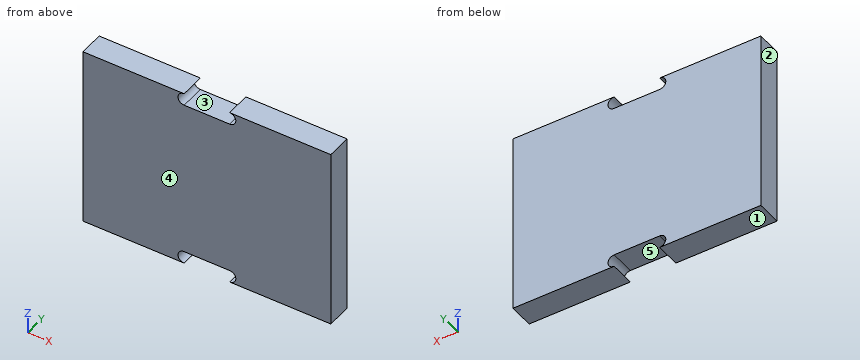
```python
from build123d import *

# Parameters (mm, degrees)
BOSS_EXTRUDE1_DEPTH = 6


with BuildPart() as part:
    # Sketch1 → Boss-Extrude1 (new body)
    with BuildSketch(Plane(origin=(0, 0, 0), x_dir=(1, 0, 0), z_dir=(0, 1, 0))):
        with BuildLine():
            Line((-30, 0), (-30, 22.2))
            Line((-30, 22.2), (-5.5, 22.2))
            ThreePointArc((-5.5, 22.2), (-7, 20.7), (-5.5, 19.2))
            Line((-5.5, 19.2), (0, 19.2))
            Line((0, 19.2), (5.5, 19.2))
            ThreePointArc((5.5, 19.2), (7, 20.7), (5.5, 22.2))
            Line((5.5, 22.2), (30, 22.2))
            Line((30, 22.2), (30, 0))
            Line((30, 0), (30, -22.2))
            Line((30, -22.2), (5.5, -22.2))
            ThreePointArc((5.5, -22.2), (7, -20.7), (5.5, -19.2))
            Line((5.5, -19.2), (0, -19.2))
            Line((0, -19.2), (-5.5, -19.2))
            ThreePointArc((-5.5, -19.2), (-7, -20.7), (-5.5, -22.2))
            Line((-5.5, -22.2), (-30, -22.2))
            Line((-30, -22.2), (-30, 0))
        make_face()
    extrude(amount=BOSS_EXTRUDE1_DEPTH)


solid = part.part
```
CAD build for the part. Positions are in the model's coordinates, mm. Face numbers are marked on the shaded views. A direction names the side the tool comes from. Coordinates: 2 decimals unless noted, no trailing zeros. Loops run counter-clockwise (first coordinate to the right, second up) from the corner with the lowest first, then second, coordinate; pieces in that order, holes last. Notation, with made-up numbers: (84, -16) - (101, -16) arc R16 cw to (101, -4) - close; hole circle Ø4 at (15.25, -34.75). An arc over 180 degrees is marked (long way). Return JSON: item names as keys, results as strings.
1. Drop flat-ended pins along their axis: pin 1 (1.5 mm diameter, centred on x = 2, z = 6.5, fed in from -Y); pin 2 (2 mm diameter, centred on x = 0, y = 2, fed in from +Z). Give the stop position or say it passes through.
Result:
{"pin 1": "stops at y = 0", "pin 2": "stops at z = 19.2"}
2. Probe L1, parallel to X at y = 0.55, z = 20.5; L2, parallel to Z at x = 6.5, y = 3.1; L3, parallel to Z at x = 3, y = 4.45. List the from-to ranges inside material, lowest first. Write a range as from..to.
Result:
{"L1": "x = -30..-6.99, 6.99..30", "L2": "z = -22.2..-21.82, -19.58..19.58, 21.82..22.2", "L3": "z = -19.2..19.2"}
3. Band-saw the part on A-A (z = 20.7). Give the cut face in (x, y).
Result:
{"outline": "(-30, 0) - (-7, 0) - (-7, 6) - (-30, 6) - close; (7, 0) - (30, 0) - (30, 6) - (7, 6) - close"}
4. Band-saw the part on C-C (x = 1.5). Give the cut face in (y, z).
Result:
{"outline": "(0, -19.2) - (6, -19.2) - (6, 19.2) - (0, 19.2) - close"}
5. 3-axis set-ups, long thin cutter, end or side, ignore diameter. For the marked faces 4 and 5: which of +Z, -Z, +X, -X, +Y, -Y reach the whole face in a straight line?
Result:
{"face 4": "+Z, -Z, +X, -X, -Y", "face 5": "-Z, +Y, -Y"}
6. Band-saw the part on B-B (y = 2.1). Give the cut face in (x, z), and give its area (3 significant figures).
Result:
{"outline": "(-30, -22.2) - (-5.5, -22.2) arc R1.5 cw to (-5.5, -19.2) - (5.5, -19.2) arc R1.5 cw to (5.5, -22.2) - (30, -22.2) - (30, 22.2) - (5.5, 22.2) arc R1.5 cw to (5.5, 19.2) - (-5.5, 19.2) arc R1.5 cw to (-5.5, 22.2) - (-30, 22.2) - close", "area": "2,580 mm2"}
7. Mould opens along X. For the marked faces 1, 2 and 3 say: released by +X, released by -X, zero draft, split by the parting line, or undercut.
Result:
{"face 1": "zero draft", "face 2": "released by -X", "face 3": "undercut"}
